Geometry: see drawing. Coordinates: mm, zero at the bounding-box minimum. A direction names the side the tool comes from. Round coordinates to 2 decimals unless told otherwise and drop trailing zeros. Loops run counter-clockwise (first coordinate to the right, second up) from the corner with the lowest first, then second, coordinate; pieces in that order, holes last. Notation, with made-up numbers: (26, 23.25) - (59, 23.25) arc R25 cw to (59, 45.25) - close; hole circle Ø6 at (23, 86). An arc over 180 degrees is marked (long way). Use CSV: the item, a comma, the result in double quotes. Start each with the question number.
1. Cut plane B-B (x = 50.8). Return loops of the section in (y, z).
2. Material intervals for probe 1 along X at (y, z) = (43.5, 39); probe 2 along Y at (x, z) = (23, 28.5) (1 decimal); probe 3 along X at (y, z) = (85.5, 4) (1 decimal), sorted ascending. Write a range as from..to.
3. Cut plane A-A (z = 29.21). Return loops of the section in (x, y), and give its area (3 significant figures).
4. Cut plane C-C (y = 38). Return loops of the section in (x, z) (1 decimal).
5. Cut plane D-D (x = 95). Return loops of the section in (y, z).
6. Pull-direction query (X, two-part tool) for the marked faces 4, 5, 6 and 7; classes: +X half, -X half, draft (parallel to the pull), parting line (faces both ways), or undercut.
7. Access query for the marked faces 1, 2 and 3. Directions: +Z, -Z, +X, -X, +Y, -Y. A direction counts if a zero-diameter tool reaches every point of the face in a straight line with its end or side. Return the directions, or none.
8. Pin query (flat end, axial travel): P1, Ø3, axis at y = 110.5, z = 20, coming from the -X side; P2, Ø4, axis at x = 26, z = 38.5, coming from the +Y side (1 decimal); P3, Ø2, axis at y = 115, z = 26.5, coming from the +X side. Return the tip coordinate at first contact, or that it passes through.
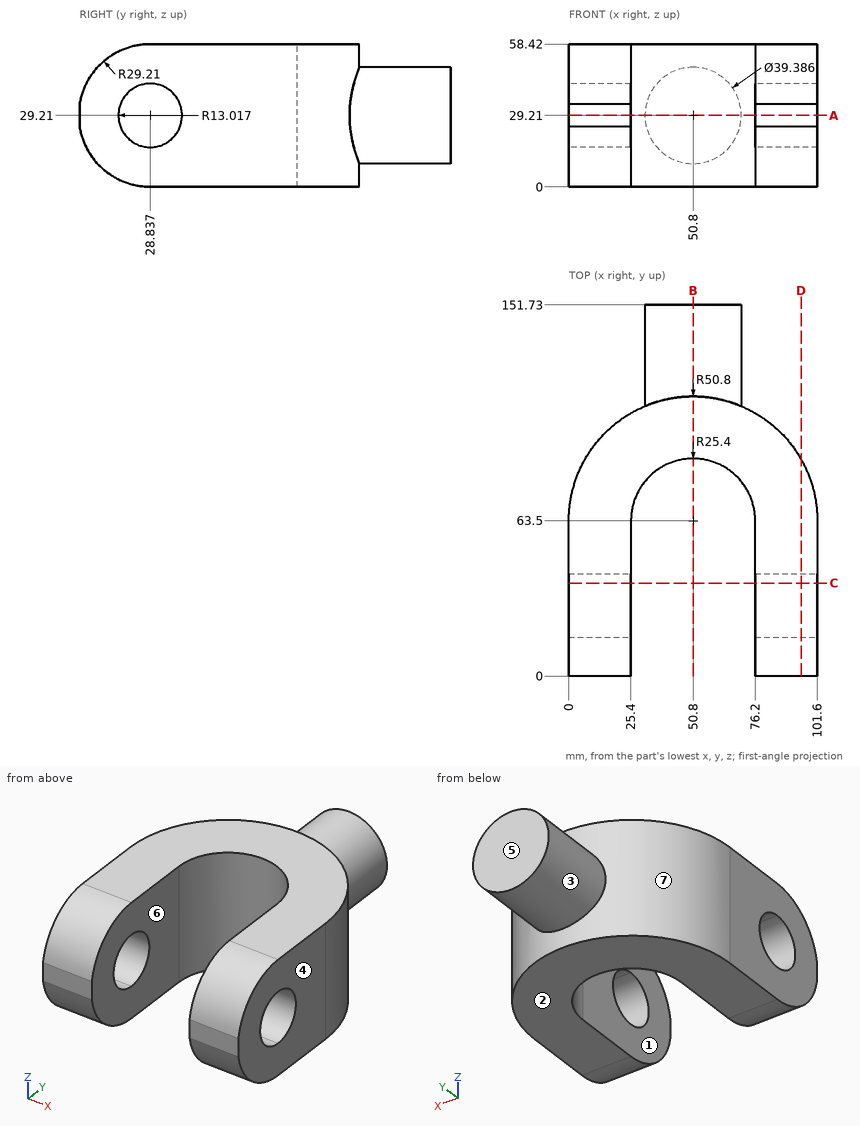
Established:
1,outline,"(88.9, 0) - (114.3, 0) - (114.3, 9.52) - (151.73, 9.52) - (151.73, 48.9) - (114.3, 48.9) - (114.3, 58.42) - (88.9, 58.42) - close"
2,probe 1,"x = 0..25.4, 76.2..101.6"
2,probe 2,"y = 0..15.8, 41.8..106"
2,probe 3,"x = 5..38.1, 63.5..96.6"
3,outline,"(0, 0) - (25.4, 0) - (25.4, 15.82) - (0, 15.82) - close; (0, 41.85) - (25.4, 41.85) - (25.4, 63.5) arc R25.4 cw to (76.2, 63.5) - (76.2, 41.85) - (101.6, 41.85) - (101.6, 63.5) arc R50.8 ccw to (70.49, 110.33) - (70.49, 151.73) - (31.11, 151.73) - (31.11, 110.33) arc R50.8 ccw to (0, 63.5) - close; (76.2, 0) - (101.6, 0) - (101.6, 15.82) - (76.2, 15.82) - close"
3,area,"6,470 mm2"
4,outline,"(0, 0) - (25.4, 0) - (25.4, 20) - (0, 20) - close; (0, 38.5) - (25.4, 38.5) - (25.4, 58.4) - (0, 58.4) - close; (76.2, 0) - (101.6, 0) - (101.6, 20) - (76.2, 20) - close; (76.2, 38.5) - (101.6, 38.5) - (101.6, 58.4) - (76.2, 58.4) - close"
5,outline,"(0, 24.56) arc R29.21 ccw to (28.84, 0) - (88.54, 0) - (88.54, 58.42) - (28.84, 58.42) arc R29.21 ccw to (0, 33.86) - close; hole circle Ø26.03 at (28.84, 29.21)"
6,face 4,"+X half"
6,face 5,"draft"
6,face 6,"undercut"
6,face 7,"parting line"
7,face 1,"+Z, -Z, -Y"
7,face 2,"-Z, +X, -X, +Y, -Y"
7,face 3,"+Y"
8,P1,"stops at x = 28.21"
8,P2,"stops at y = 108.9"
8,P3,"stops at x = 70.42"
